from build123d import *

# Parameters (mm, degrees)
F0_R     = 62.5
F0_R_2   = 2.5
F0_R_3   = 36
F1_DEPTH = 3
F0_R_4   = 7.5
F2_DEPTH = 5


with BuildPart() as f1:
    # F0 (on Right) → F1 (new body)
    with BuildSketch(Plane.YZ):
        Circle(F0_R)
        with Locations((0, -56.5)):
            Circle(F0_R_2, mode=Mode.SUBTRACT)
        with Locations((-56.5, 0)):
            Circle(F0_R_2, mode=Mode.SUBTRACT)
        Circle(F0_R_3, mode=Mode.SUBTRACT)
        with Locations((56.5, 0)):
            Circle(F0_R_2, mode=Mode.SUBTRACT)
        with Locations((0, 56.5)):
            Circle(F0_R_2, mode=Mode.SUBTRACT)
    extrude(amount=F1_DEPTH)

    # F0 (on Right) → F2 (join)
    with BuildSketch(Plane.YZ):
        Circle(F0_R)
        with Locations((0, -56.5)):
            Circle(F0_R_2, mode=Mode.SUBTRACT)
        with Locations((-56.5, 0)):
            Circle(F0_R_2, mode=Mode.SUBTRACT)
        Circle(F0_R_3, mode=Mode.SUBTRACT)
        with Locations((56.5, 0)):
            Circle(F0_R_2, mode=Mode.SUBTRACT)
        with Locations((0, 56.5)):
            Circle(F0_R_2, mode=Mode.SUBTRACT)
        Circle(F0_R_3)
        with Locations((0, -20)):
            Circle(F0_R_2, mode=Mode.SUBTRACT)
        with Locations((-20, 0)):
            Circle(F0_R_2, mode=Mode.SUBTRACT)
        Circle(F0_R_4, mode=Mode.SUBTRACT)
        with Locations((20, 0)):
            Circle(F0_R_2, mode=Mode.SUBTRACT)
        with Locations((0, 20)):
            Circle(F0_R_2, mode=Mode.SUBTRACT)
    extrude(amount=-F2_DEPTH)


solid = f1.part
Verification items for the finished model (mm, model axes). A direction names the side the tool comes from. Give positions to 0.01 mm unless a question says otherwise; leave off trailing zeros. Loops run counter-clockwise (first coordinate to the right, second up) from the corner with the lowest first, then second, coordinate; pieces in that order, holes last. Notation, with made-up numbers: (-11, 60.25) - (33, 60.25) arc R22 ccw to (33, 67.25) - close; hole circle Ø1 at (69.5, 24.5). An arc over 180 degrees is marked (long way). Write item = value, one per line. Start each with the question number.
Q1. Depth check by flat-ended pin: P1, Ø6.5, axis at y = 0, z = 20, coming from the +X side; P2, Ø2, axis at x = 0.5, z = 31, coming from the +Y side; P3, Ø2, axis at x = -0.5, z = -19.5, coming from the -Y side. Enter the tip coordinate at first touch or a pass-through.
Q2. Cross-section at A-A, the plane x = -2.75. State how many separate pieces and enclosed holes the cut face has, and give its area (3 significant figures).
Q3. Thickness scan on line 1 (Z direction, x = 0.5, y = 0); line 2 (Z direction, x = -2, y = -6); line 3 (X direction, y = 3, z = -24). Record the ranges inside material, lowest first.
Q4. Cross-section at B-B, the plane y = 56.5. Enter the section's corners in (x, z).
Q5. Tool access check on faces 4 (the face through (1.479, -4.686, 35.694)), 5 (the face through (-1.06, -0.54, 54.06)). Record the directions out of +Z, -Z, +X, -X, +Y, -Y that give a thin tool (end or side, any length) a straight path to the whole face; none if there is none.
Q6. Cross-section at D-D, the plane z = -13.5. Enter the section's corners in (x, y).
Q7. Mould release check, pull along Z, two halves, no side actions. Record for faces 1 (the face through (3, 27, -27)), 2 (the face through (-0.94, -62.44, 2.75)), 3 (the face through (-2.46, -0.33, 22.48)): released by +Z, released by -Z, zero draft, split by the parting line, or undercut.
Answer key:
q1.P1 = 0
q1.P2 = 54.83
q1.P3 = -59.7
q2.separate_pieces = 1
q2.enclosed_holes = 9
q2.area = 11,900 mm^2
q3.line_1 = -62.5 to -59, -54 to -36, 36 to 54, 59 to 62.5
q3.line_2 = -62.21 to -4.5, 4.5 to 62.21
q3.line_3 = -5 to 0
q4.outline = (-5, -26.72) - (3, -26.72) - (3, -2.5) - (-5, -2.5) - close; (-5, 2.5) - (3, 2.5) - (3, 26.72) - (-5, 26.72) - close
q5.face_4 = +X
q5.face_5 = +X, -X
q6.outline = (-5, -61.02) - (3, -61.02) - (3, -33.37) - (0, -33.37) - (0, 33.37) - (3, 33.37) - (3, 61.02) - (-5, 61.02) - close
q7.face_1 = zero draft
q7.face_2 = split by the parting line
q7.face_3 = undercut
